The model under review builds one solid part; all positions refer to its coordinate system, in mm. Face numbers are marked on the shaded views. A direction names the side the tool comes from. Round coordinates to 2 decimals unless told otherwise and drop trailing zeros. Loops run counter-clockwise (first coordinate to the right, second up) from the corner with the lowest first, then second, coordinate; pieces in that order, holes last. Notation, with made-up numbers: M -11.75,28.25 L 20.25,28.25 A18 ccw 20.25,33.25 Z; hole C 44,9.25 d8. An arc over 180 degrees is marked long. Return JSON: item names as keys, results as strings. Group by question number.
Q1. Consider section A-A (y = 0). State the section outline as (x, z) points, and give its area (3 significant figures).
Q2. Draft analysis for pull direction Z (two halves, no side actions). For the marked faces 4, 5 and 6, state which applies: pulls with the +Z half, pulls with the -Z half, needs draft (parallel to the pull), parting line crosses it, or undercut.
Q3. Consider section C-C (y = -8.75). State the section outline as (x, z) points, and give its area (3 significant figures).
Q4. For the marked faces 1, 2 and 3, list the 3-axis set-ups (+Z, -Z, +X, -X, +Y, -Y) from which the entire face can be reached by the end or side of a thin tool; tool diameter is ignored.
Q5. Consider section B-B (z = 23.5). State the section outline as (x, y) points, and give its area (3 significant figures).
Q6. Consider section D-D (z = 14). State the section outline as (x, y) points.
Q7. Clearance check with flat-ended pins moving along their axes: pin 1 Ø12.5 at (x, z) = (-2.5, 28) entering from +Y; pin 2 Ø12.5 at (x, z) = (-3, 25.5) entering from -Y; pin 3 Ø8 at (x, z) = (-8, 50.5) entering from -Y. State where each tip first meets the part, or that it passes through.
Q8. To check wall thickness, follow line 1 along Z through (x, y) = (-5.5, 0); line 2 along Y through (x, z) = (-8, 21.5); line 3 along Z through (x, y) = (-1.25, 11.5). State the ranges of each line that lie inside material, in increasing order.
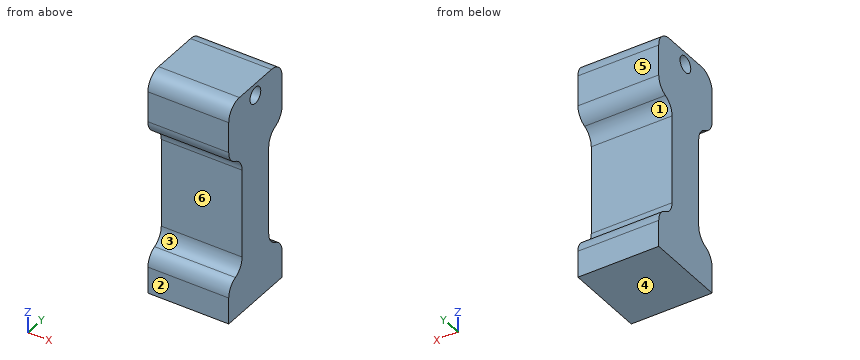
from build123d import *

# Parameters (mm, degrees)
F0_W     = 25.4
F0_H     = 25.4
F1_DEPTH = 69.85
F2_R     = 2.5527
F3_DEPTH = 25.4
F4_R     = 5.08
F5_W     = 6.35
F5_H     = 38.1
F6_DEPTH = 25.4
F7_R     = 5.08
F8_R     = 5.08


with BuildPart() as f1:
    # F0 (on Top) → F1 (new body)
    with BuildSketch(Plane.XY):
        Rectangle(F0_W, F0_H)
    extrude(amount=F1_DEPTH)

    # F2 (on face) → F3 (cut)
    with BuildSketch(Plane.YZ.offset(12.7)):
        with Locations((0, 66.0527)):
            Circle(F2_R)
    extrude(amount=-F3_DEPTH, mode=Mode.SUBTRACT)

    # F4
    f4_edges = [f1.edges().sort_by_distance(p)[0] for p in [
        (0, -12.7, 69.85),
        (0, 12.7, 69.85),
    ]]
    fillet(f4_edges, radius=F4_R)

    # F5 (on face) → F6 (cut)
    with BuildSketch(Plane.YZ.offset(12.7)):
        with Locations((-9.525, 31.75)):
            Rectangle(F5_W, F5_H)
        with Locations((9.525, 31.75)):
            Rectangle(F5_W, F5_H)
    extrude(amount=-F6_DEPTH, mode=Mode.SUBTRACT)

    # F7
    f7_edges = [f1.edges().sort_by_distance(p)[0] for p in [
        (0, 6.35, 50.8),
        (0, 6.35, 12.7),
        (0, -6.35, 50.8),
        (0, -6.35, 12.7),
    ]]
    fillet(f7_edges, radius=F7_R)

    # F8
    f8_edges = [f1.edges().sort_by_distance(p)[0] for p in [
        (0, -12.7, 12.7),
        (0, -12.7, 50.8),
        (0, 12.7, 12.7),
        (0, 12.7, 50.8),
    ]]
    fillet(f8_edges, radius=F8_R)


solid = f1.part
Values:
{
 "1": {"outline": "M -12.7,0 L 12.7,0 L 12.7,63.5 L -12.7,63.5 Z; M -12.7,68.61 L 12.7,68.61 L 12.7,69.85 L -12.7,69.85 Z", "area": "1,640 mm2"},
 "2": {"face 4": "pulls with the -Z half", "face 5": "needs draft", "face 6": "undercut"},
 "3": {"outline": "M -12.7,0 L 12.7,0 L 12.7,13.46 L -12.7,13.46 Z; M -12.7,50.04 L 12.7,50.04 L 12.7,69.72 L -12.7,69.72 Z", "area": "842 mm2"},
 "4": {"face 1": "+X, -X, +Y", "face 2": "+Z, -Z, +X, -X, -Y", "face 3": "+X, -X, -Y"},
 "5": {"outline": "M -12.7,-6.35 L 12.7,-6.35 L 12.7,6.35 L -12.7,6.35 Z", "area": "323 mm2"},
 "6": {"outline": "M -12.7,-8.04 L 12.7,-8.04 L 12.7,8.04 L -12.7,8.04 Z"},
 "7": {"pin 1": "stops at y = 6.35", "pin 2": "stops at y = -6.35", "pin 3": "stops at y = -12.66"},
 "8": {"line 1": "z = 0 to 63.5, 68.61 to 69.85", "line 2": "y = -6.35 to 6.35", "line 3": "z = 0 to 11.64, 51.86 to 68.05"}
}
